Source: CAD feature listing. Evaluate the final solid. Frame: model axes, mm. A direction names the side the tool comes from. Give positions to 0.01 mm unless a question says otherwise; leave off trailing zeros. Order: outer loops, then holes, each group sorted by start corner. A loop starts at its lowest first (then second) coordinate and runs counter-clockwise, first axis right, second up.
```python
from build123d import *

# Parameters (mm, degrees)
SKETCH2_R          = 2.65
CUT_EXTRUDE1_DEPTH = 10


with BuildPart() as part:
    # Sketch1 → Revolve1 (revolve)
    with BuildSketch(Plane.XY, mode=Mode.PRIVATE) as revolve1_sk:
        Polygon((5.75, 10), (17.2, 10), (17.2, 0), (16.5, 0), (16.5, 8), (5.75, 8), align=None)
    revolve(revolve1_sk.sketch.rotate(Axis((0, -9.26010101, 0), (0, 1, 0)), 90), axis=Axis((0, -9.26010101, 0), (0, 1, 0)))

    # Sketch2 → Cut-Extrude1 (cut)
    with BuildSketch(Plane.XZ.offset(-8)):
        with Locations(Location((-11, 0, 0), (0, 0, 270))):
            Circle(SKETCH2_R)
        with Locations(Location((11, 0, 0), (0, 0, 270))):
            Circle(SKETCH2_R)
    extrude(amount=-CUT_EXTRUDE1_DEPTH, mode=Mode.SUBTRACT)


solid = part.part
```
1) Section query D-D, the plane z = -4.5. Return the cut outline in (x, y).
Report:
outline: (-16.6, 0) - (-15.87, 0) - (-15.87, 8) - (-3.58, 8) - (-3.58, 10) - (-16.6, 10) - close; (3.58, 8) - (15.87, 8) - (15.87, 0) - (16.6, 0) - (16.6, 10) - (3.58, 10) - close
2) Reachability of faces 5 (the flat face through (7, 8, 0)), 6 (the cylindrical face through (-5.7, 9.01, 0.75)) from +Z, -Z, +X, -X, +Y, -Y: full face, straight path, thin tool, end or side. Return the list, or none.
Report:
face 5: -Y
face 6: +Y, -Y
3) Pin query (flat end, axial travel): pin 1 (4 mm diameter, centred on y = 6, z = 12.5, fed in from +X); pin 2 (1 mm diameter, centred on x = 4, y = 9, fed in from +Z); pin 3 (8 mm diameter, centred on x = 7, z = -8.5, fed in from -Y). Return the tip coordinate at first contact, or that it passes through.
Report:
pin 1: stops at x = 13.62
pin 2: stops at z = 16.84
pin 3: stops at y = 8
4) Section query B-B, the plane x = 11. Return the cut outline in (y, z), and give its area (3 significant figures).
Report:
outline: (0, -13.22) - (10, -13.22) - (10, -2.65) - (8, -2.65) - (8, -12.3) - (0, -12.3) - close; (0, 12.3) - (8, 12.3) - (8, 2.65) - (10, 2.65) - (10, 13.22) - (0, 13.22) - close
area: 57.1 mm2
5) Material intervals for L1, parallel to X at y = 8.75, z = 0; L2, parallel to Y at x = -8.5, z = 1.5; L3, parallel to Z at x = -4, y = 2.25, sorted ascending.
Report:
L1: x = -17.2 to -13.65, -8.35 to -5.75, 5.75 to 8.35, 13.65 to 17.2
L2: y = 8 to 10
L3: z = -16.73 to -16.01, 16.01 to 16.73
6) Draft query along X for faces 1 (the cylindrical face through (8.41, 8.99, 0.57)), 2 (the cylindrical face through (-13.59, 8.99, 0.57)), 3 (the cylindrical face through (-0.756, 4.93, 17.183)), 4 (the flat face through (7, 10, 0)). Return one class per face: +X half, -X half, draft (parallel to the pull), parting line (faces both ways), or undercut.
Report:
face 1: undercut
face 2: undercut
face 3: parting line
face 4: draft
7) Section query A-A, the plane z = 0. Return the cut outline in (x, y), and give its area (3 significant figures).
Report:
outline: (-17.2, 0) - (-16.5, 0) - (-16.5, 8) - (-13.65, 8) - (-13.65, 10) - (-17.2, 10) - close; (-8.35, 8) - (-5.75, 8) - (-5.75, 10) - (-8.35, 10) - close; (5.75, 8) - (8.35, 8) - (8.35, 10) - (5.75, 10) - close; (13.65, 8) - (16.5, 8) - (16.5, 0) - (17.2, 0) - (17.2, 10) - (13.65, 10) - close
area: 35.8 mm2
8) Section query C-C, the plane y = 8.5. Return the cut outline in (x, z).
Report:
outline: circle Ø34.4 at (0, 0); hole circle Ø5.3 at (-11, 0); hole circle Ø11.5 at (0, 0); hole circle Ø5.3 at (11, 0)
